Read the model definition and answer for the solid it produces. Units are mm, in the model's axes. A direction names the side the tool comes from. Give positions to 0.01 mm unless a question says otherwise; leave off trailing zeros. Order: outer loops, then holes, each group sorted by start corner. A loop starts at its lowest first (then second) coordinate and runs counter-clockwise, first axis right, second up. Notation, with made-up numbers: (49.5, 31) - (70.5, 31) arc R19 ccw to (70.5, 44) - close; hole circle Ø11 at (89.5, 29.5). An arc over 180 degrees is marked (long way). Write each question's results on one line, items separated by ' | '. Start each with the question number.
Q1. For a pull along Y with two mould halves and no side action, classify faces 4 (the face through (-108.842, 152.688, 58.411)), 5 (the face through (-49, 145, 0)), 6 (the face through (-49, 145, 18)) as +Y half, -Y half, draft (parallel to the pull), parting line (faces both ways), or undercut.
Q2. Find the intervals of material crossed by line 1 along Y through (x, z) = (-115, 36.5); line 2 along Z through (x, y) = (-28, 170); line 3 along Y through (x, z) = (-109.5, 40), in increasing order. Write a range as from..to.
Q3. A tool of negligible diameter and unlimited length cuts with its end or side. For faces 1 (the face through (-117.3, 166.2, 18)), 2 (the face through (-115, 163.1, 33.8)), 3 (the face through (-43.51, 150.43, 28.59)), from which of +Z, -Z, +X, -X, +Y, -Y can it reach the whole face along a straight path? Write none if from no direction.
Q4. Find section B-B on y = 177.5. Give the vertices of the cut face in (x, z).
Q5. Find section A-A on z = 43.5. Count the separate pieces of the cut face and the enclosed holes in it, and give its area (3 significant figures).
Q6. Flat-ended cylindrical pins translate along their axes: P1, Ø2, axis at x = -47, z = 24.5, coming from the -Y side; P2, Ø3, axis at x = -51.5, z = 27.5, coming from the -Y side; P3, Ø1.5, axis at y = 132.5, z = 39, coming from the -X side; P4, Ø10, axis at y = 142, z = 52, coming from the -X side. Find the tip coordinate at first contact, or state that the pin passes through.
Q7. Find section C-C on x = -25. Give the vertices of the cut face in (y, z).
Q8. Find section D-D on y = 192.5. Give the vertices of the cut face in (x, z), and give its area (3 significant figures).
from build123d import *

# Parameters (mm, degrees)
BOX035_W                  = 6
BOX035_H                  = 15
BOX035_DEPTH              = 3
CYLINDER018_R             = 2
CYLINDER018_DEPTH         = 50
BOX_W                     = 15
BOX_H                     = 15
BOX_DEPTH                 = 58
CUT051_PLACEMENT_ANGLE    = 60
CUT052_PLACEMENT_ANGLE    = 60
BOX044_W                  = 80
BOX044_H                  = 5
BOX044_DEPTH              = 58
BOX045_W                  = 80
BOX045_H                  = 90
BOX045_DEPTH              = 4
FUSION090_PLACEMENT_ANGLE = 120


with BuildPart() as nut_hole:
    # Box035 → Box035 (new body)
    with BuildSketch(Plane(origin=(-8.5, 5, 15), x_dir=(1, 0, 0), z_dir=(0, 0, 1))):
        with Locations((3, 7.5)):
            Rectangle(BOX035_W, BOX035_H)
    extrude(amount=BOX035_DEPTH)


with BuildPart() as cylinder:
    # Cylinder018 → Cylinder018 (new body)
    with BuildSketch(Plane(origin=(-5.5, 12, 0), x_dir=(1, 0, 0), z_dir=(0, 0, 1))):
        Circle(CYLINDER018_R)
    extrude(amount=CYLINDER018_DEPTH)


with BuildPart() as cut:
    # Box → Box (new body)
    with BuildSketch(Plane(origin=(-13, 5, 0), x_dir=(1, 0, 0), z_dir=(0, 0, 1))):
        with Locations((7.5, 7.5)):
            Rectangle(BOX_W, BOX_H)
    extrude(amount=BOX_DEPTH)

    # Cut: cut Cylinder
    add(cylinder.part, mode=Mode.SUBTRACT)


with BuildPart() as cut051:
    # Cut051 base: copy of Cut
    add(cut.part)

    # Cut051: cut Nut hole
    add(nut_hole.part, mode=Mode.SUBTRACT)


with BuildPart() as cut051_1:
    # Cut051 placement: moved
    add(cut051.part.moved(Location((-102.160254, 163.841633, 0))).rotate(Axis((-102.160254, 163.841633, 0), (0, 0, 1)), CUT051_PLACEMENT_ANGLE))


with BuildPart() as cut052:
    # Cut052 base: copy of Cut
    add(cut.part)

    # Cut052: cut Nut hole
    add(nut_hole.part, mode=Mode.SUBTRACT)


with BuildPart() as cut052_1:
    # Cut052 placement: moved
    add(cut052.part.moved(Location((-33.77171, 142.497283, 0))).rotate(Axis((-33.77171, 142.497283, 0), (0, 0, 1)), CUT052_PLACEMENT_ANGLE))


with BuildPart() as cube006:
    # Box044 → Box044 (new body)
    with BuildSketch(Plane(origin=(-35, 0, 0), x_dir=(1, 0, 0), z_dir=(0, 0, 1))):
        with Locations((40, 2.5)):
            Rectangle(BOX044_W, BOX044_H)
    extrude(amount=BOX044_DEPTH)


with BuildPart() as fusion092:
    # Box045 → Box045 (new body)
    with BuildSketch(Plane(origin=(-35, 0, 58), x_dir=(1, 0, 0), z_dir=(0, 0, 1))):
        with Locations((40, 45)):
            Rectangle(BOX045_W, BOX045_H)
    extrude(amount=BOX045_DEPTH)

    # Fusion090: union Cube006
    add(cube006.part)


with BuildPart() as fusion092_1:
    # Fusion090 placement: moved
    add(fusion092.part.moved(Location((-107.811, 204.054, 0))).rotate(Axis((-107.811, 204.054, 0), (0, 0, -1)), FUSION090_PLACEMENT_ANGLE))

    # Fusion092: union Cut051, Cut052
    add(cut051_1.part)
    add(cut052_1.part)


solid = fusion092_1.part
Working result:
1) face 4: -Y half | face 5: draft | face 6: undercut
2) line 1: 156.24..163.1, 167.06..173.56, 181.6..191.6 | line 2: 58..62 | line 3: 161.13..170.39, 191.13..201.13
3) face 1: none | face 2: -Z | face 3: -Z, +X, +Y
4) outline: (-123.14, 0) - (-117.37, 0) - (-117.37, 58) - (-19.22, 58) - (-19.22, 62) - (-123.14, 62) - close
5) separate pieces: 2 | enclosed holes: 2 | area: 825 mm²
6) P1: y = 134.55 | P2: y = 136.86 | P3: through | P4: x = -57.59
7) outline: (167.49, 58) - (196.66, 58) - (196.66, 62) - (167.49, 62) - close
8) outline: (-114.48, 0) - (-108.71, 0) - (-108.71, 58) - (-17.8, 58) - (-17.8, 62) - (-114.48, 62) - close | area: 722 mm²
